from build123d import *

# Parameters (mm, degrees)
F0_W     = 38.1
F0_H     = 76.2
F0_W_2   = 101.6
F0_W_3   = 1.5875
F0_H_2   = 19.05
F1_DEPTH = 25.4


with BuildPart() as f1:
    # F0 (on Top) → F1 (new body)
    with BuildSketch(Plane.XY):
        Polygon((88.9, 38.1), (50.8, 38.1), (50.8, 9.525), (50.8, -9.525), (50.8, -38.1), (88.9, -38.1), (127, -38.1), (127, 38.1), align=None)
        with Locations((69.85, 76.2)):
            Rectangle(F0_W, F0_H)
        with Locations((0, 76.2)):
            Rectangle(F0_W_2, F0_H)
        Polygon((-50.8, 9.525), (-50.8, 38.1), (-88.9, 38.1), (-127, 38.1), (-127, -38.1), (-88.9, -38.1), (-50.8, -38.1), (-50.8, -9.525), align=None)
        with Locations((-69.85, 76.2)):
            Rectangle(F0_W, F0_H)
        with Locations((0, 152.4)):
            Rectangle(F0_W_2, F0_H)
        with Locations((127.79375, 0)):
            Rectangle(F0_W_3, F0_H)
        with BuildLine():
            Line((-50.8, 190.5), (50.8, 190.5))
            Line((50.8, 190.5), (50.8, 215.9))
            ThreePointArc((50.8, 215.9), (47.0802561211, 224.8802561211), (38.1, 228.6))
            Line((38.1, 228.6), (-38.1, 228.6))
            ThreePointArc((-38.1, 228.6), (-47.0802561211, 224.8802561211), (-50.8, 215.9))
            Line((-50.8, 215.9), (-50.8, 190.5))
        make_face()
        with Locations((-127.79375, 0)):
            Rectangle(F0_W_3, F0_H)
        with Locations((0, -76.2)):
            Rectangle(F0_W_2, F0_H)
        with Locations((69.85, -76.2)):
            Rectangle(F0_W, F0_H)
        Polygon((204.7875, 38.1), (128.5875, 38.1), (128.5875, -38.1), (204.7875, -38.1), (204.7875, -9.525), (204.7875, 9.525), align=None)
        with Locations((-69.85, -76.2)):
            Rectangle(F0_W, F0_H)
        Polygon((-128.5875, -38.1), (-128.5875, 38.1), (-204.7875, 38.1), (-204.7875, 9.525), (-204.7875, -9.525), (-204.7875, -38.1), align=None)
        with Locations((205.58125, 0)):
            Rectangle(F0_W_3, F0_H_2)
        with Locations((-205.58125, 0)):
            Rectangle(F0_W_3, F0_H_2)
        Polygon((50.8, 9.525), (50.8, 38.1), (-50.8, 38.1), (-50.8, 9.525), (-49.2125, 9.525), (-49.2125, -9.525), (-50.8, -9.525), (-50.8, -38.1), (50.8, -38.1), (50.8, -9.525), (49.2125, -9.525), (49.2125, 9.525), align=None)
    extrude(amount=F1_DEPTH)


solid = f1.part
Could you check a few things on this model? Use its own coordinates, in mm. A direction names the side the tool comes from. Round coordinates to 2 decimals unless told otherwise and drop trailing zeros. Order: outer loops, then holes, each group sorted by start corner. A loop starts at its lowest first (then second) coordinate and runs counter-clockwise, first axis right, second up.
Q1. Thinking about a two-plate mould opening in X: for faces 1 (the face through (50.8, 0, 13)), 2 (the face through (146, -38.1, 13)), 3 (the face through (-206.375, 0, 13)), 4 (the face through (-50.8, 0, 13)), which applies, released by +X, released by -X, zero draft, split by the parting line, or undercut?
Geometry says:
face 1: undercut
face 2: zero draft
face 3: released by -X
face 4: undercut
Q2. Imagine slicing it at C-C, the plane x = -178. List the corners of the cut face in (y, z) for me.
Geometry says:
outline: (-38.1, 0) - (38.1, 0) - (38.1, 25.4) - (-38.1, 25.4) - close
Q3. Imagine slicing it at B-B, the plane y = 195. List the corners of the cut face in (x, z) for me.
Geometry says:
outline: (-50.8, 0) - (50.8, 0) - (50.8, 25.4) - (-50.8, 25.4) - close
Q4. I'm going to push flat-ended pins straight in: P1, Ø1.3, axis at x = 205.5, z = 18, coming from the -Y side (3 decimals); P2, Ø10, axis at x = -146, z = 3.5, coming from the -Y side; P3, Ø12, axis at x = 59, z = 9.5, coming from the +Y side; P4, Ø1.5, axis at x = -21, y = 75.5, coming from the -Z side. Where does each tip first touch, or does it pass through?
Geometry says:
P1: stops at y = -9.525
P2: stops at y = -38.1
P3: stops at y = 114.3
P4: stops at z = 0
Q5. Which directions (+Z, -Z, +X, -X, +Y, -Y) give clear straight access to the entire face, cutting with the end or side of a thin tool? Please do faces 5 (the face through (-3, 21, 25.4)), 6 (the face through (88.9, -77, 13)), 7 (the face through (148, 38.1, 13)), 8 (the face through (-50.8, 166, 13)), 9 (the face through (-204.788, -24, 13)).
Geometry says:
face 5: +Z, +X, -X, +Y, -Y
face 6: +Z, -Z, +X, -Y
face 7: +Z, -Z, +X, +Y
face 8: +Z, -Z, -X, +Y
face 9: +Z, -Z, -X, -Y
Q6. Please list where these lines run through material, in increasing order: probe 1 along X at (y, z) = (141.5, 16.5); probe 2 along Y at (x, z) = (107, 14); probe 3 along X at (y, z) = (-63.5, 11.5).
Geometry says:
probe 1: x = -50.8 to 50.8
probe 2: y = -38.1 to 38.1
probe 3: x = -88.9 to 88.9
Q7. Imagine slicing it at A-A, the plane z = 7.75. State how many separate pieces and enclosed holes the cut face has, then the cut area to 4 significant figures.
Geometry says:
separate pieces: 1
enclosed holes: 2
area: 69,850 mm2
